from build123d import *

# Parameters (mm, degrees)
F0_R     = 3
F0_R_2   = 4.5
F0_R_3   = 11.5
F1_DEPTH = 2
F2_DEPTH = 2.5
F3_DEPTH = 6


with BuildPart() as f1:
    # F0 (on Front) → F1 (new body)
    with BuildSketch(Plane.XZ):
        Circle(F0_R)
        Circle(F0_R_2)
        Circle(F0_R, mode=Mode.SUBTRACT)
        Circle(F0_R_3)
        Circle(F0_R_2, mode=Mode.SUBTRACT)
    extrude(amount=F1_DEPTH)

    # F0 (on Front) → F2 (join)
    with BuildSketch(Plane.XZ):
        Circle(F0_R_2)
        Circle(F0_R, mode=Mode.SUBTRACT)
    extrude(amount=F2_DEPTH)

    # F0 (on Front) → F3 (join)
    with BuildSketch(Plane.XZ):
        Circle(F0_R)
    extrude(amount=F3_DEPTH)


solid = f1.part
Check sheet for the modelled part. Datum: model origin and axes. Units: mm. A direction names the side the tool comes from. Round coordinates to 2 decimals unless told otherwise and drop trailing zeros. Loops run counter-clockwise (first coordinate to the right, second up) from the corner with the lowest first, then second, coordinate; pieces in that order, holes last. Notation, with made-up numbers: (-2, 13) - (32, 13) arc R35 cw to (32, 51) - close; hole circle Ø8 at (50, -38.75). An arc over 180 degrees is marked (long way). Answer as CSV lines item,"result". Start each with the question number.
Item 1: Section check A-A (x = 0). Record the boundary of the cut face in (y, z), and give its area (3 significant figures).
Item 2: Depth check by flat-ended pin: P1, Ø4, axis at x = -6, z = -2, coming from the -Y side; P2, Ø1.5, axis at x = 5, y = -3.5, coming from the +Z side; P3, Ø2, axis at y = -1, z = -7.5, coming from the +X side; P4, Ø12, axis at x = 8.5, z = -1, coming from the +Y side. Enter the tip coordinate at first touch or a pass-through.
Item 3: Section check D-D (y = -3.75). Record the boundary of the cut face in (x, z).
Item 4: Set-up check for faces 1 (the flat face through (5, -2, 0)), 2 (the cylindrical face through (-1.5, -1, 11.4)): record each of +Z, -Z, +X, -X, +Y, -Y from which the full face is reachable in a straight line by a thin tool's end or side.
Item 5: Section check B-B (y = -1.2). Record the boundary of the cut face in (x, z), and give its area (3 significant figures).
Item 6: Section check C-C (z = -0.5). Record the boundary of the cut face in (x, y), and give its area (3 significant figures).
Item 7: Scan lines: line 1 (Y direction, x = -1, z = -7.5); line 2 (X direction, y = -0.25, z = -3); line 3 (X direction, y = -1.5, z = -8.5). Record each from-to range of solid material in increasing order. Write a range as [from, to].
Report:
1,outline,"(-6, -3) - (-2.5, -3) - (-2.5, -4.5) - (-2, -4.5) - (-2, -11.5) - (0, -11.5) - (0, 11.5) - (-2, 11.5) - (-2, 4.5) - (-2.5, 4.5) - (-2.5, 3) - (-6, 3) - close"
1,area,"71.5 mm2"
2,P1,"stops at y = -2.5"
2,P2,"passes through"
2,P3,"stops at x = 9.49"
2,P4,"stops at y = 0"
3,outline,"circle Ø6 at (0, 0)"
4,face 1,"-Y"
4,face 2,"+Y, -Y"
5,outline,"circle Ø23 at (0, 0)"
5,area,"415 mm2"
6,outline,"(-11.49, -2) - (-4.47, -2) - (-4.47, -2.5) - (-2.96, -2.5) - (-2.96, -6) - (2.96, -6) - (2.96, -2.5) - (4.47, -2.5) - (4.47, -2) - (11.49, -2) - (11.49, 0) - (-11.49, 0) - close"
6,area,"71.1 mm2"
7,line 1,"y = [-2, 0]"
7,line 2,"x = [-11.1, 11.1]"
7,line 3,"x = [-7.75, 7.75]"
